The model under review builds one solid part; all positions refer to its coordinate system, in mm. A direction names the side the tool comes from. Round coordinates to 2 decimals unless told otherwise and drop trailing zeros. Loops run counter-clockwise (first coordinate to the right, second up) from the corner with the lowest first, then second, coordinate; pieces in that order, holes last. Notation, with made-up numbers: (15, 88.25) -> (61, 88.25) arc R17 cw to (61, 104.25) -> close; hole circle Ø10 at (36.25, 16.5). An arc over 180 degrees is marked (long way). Return JSON: item names as keys, results as strings. Group by question number.
```python
from build123d import *

# Parameters (mm, degrees)
SKETCH1_R           = 3.175
BOSS_EXTRUDE1_DEPTH = 5.842
FILLET1_R           = 6.35
FILLET2_R           = 12.7


with BuildPart() as part:
    # Sketch1 → Boss-Extrude1 (new body)
    with BuildSketch(Plane.XY):
        with BuildLine():
            Line((-22.994485403, 20.272024726), (-17.997254848, 15.918288597))
            Line((-17.997254848, 15.918288597), (-17.997254848, 5.482991472))
            Line((-17.997254848, 5.482991472), (-22.994485403, 1.145618131))
            ThreePointArc((-22.994485403, 1.145618131), (-24.602923257, -1.012071311), (-25.173214286, -3.642178571))
            ThreePointArc((-25.173214286, -3.642178571), (-21.763981419, -9.270178986), (-15.197028879, -8.854978145))
            Line((-15.197028879, -8.854978145), (-1.135121582, 0.926921642))
            Line((-1.135121582, 0.926921642), (26.988693011, 0.926921642))
            Line((26.988693011, 0.926921642), (42.638100307, -8.854978145))
            ThreePointArc((42.638100307, -8.854978145), (49.205052848, -9.270178986), (52.614285714, -3.642178571))
            ThreePointArc((52.614285714, -3.642178571), (52.043994686, -1.012071311), (50.435556832, 1.145618131))
            Line((50.435556832, 1.145618131), (46.348568334, 6.363266694))
            Line((46.348568334, 6.363266694), (46.348568334, 16.798563819))
            Line((46.348568334, 16.798563819), (50.435556832, 20.272024726))
            ThreePointArc((50.435556832, 20.272024726), (51.272005862, 28.964336626), (42.638100307, 30.272621002))
            Line((42.638100307, 30.272621002), (26.988693011, 20.490721215))
            Line((26.988693011, 20.490721215), (-1.135121582, 20.490721215))
            Line((-1.135121582, 20.490721215), (-15.197028879, 30.272621002))
            ThreePointArc((-15.197028879, 30.272621002), (-23.830934433, 28.964336626), (-22.994485403, 20.272024726))
        make_face()
        with Locations((-18.823214286, -3.642178571)):
            Circle(SKETCH1_R, mode=Mode.SUBTRACT)
        with Locations((46.264285714, -3.642178571)):
            Circle(SKETCH1_R, mode=Mode.SUBTRACT)
        with Locations((-18.823214286, 25.059821429)):
            Circle(SKETCH1_R, mode=Mode.SUBTRACT)
        with Locations((46.264285714, 25.059821429)):
            Circle(SKETCH1_R, mode=Mode.SUBTRACT)
    extrude(amount=BOSS_EXTRUDE1_DEPTH)

    # Fillet1
    fillet1_edges = [part.edges().sort_by_distance(p)[0] for p in [
        (-17.997254848, 5.482991472, 2.921),
        (-17.997254848, 15.918288597, 2.921),
        (46.348568334, 16.798563819, 2.921),
        (46.348568334, 6.363266694, 2.921),
    ]]
    fillet(fillet1_edges, radius=FILLET1_R)

    # Fillet2
    fillet2_edges = [part.edges().sort_by_distance(p)[0] for p in [
        (26.988693011, 0.926921642, 2.921),
        (-1.135121582, 0.926921642, 2.921),
        (-1.135121582, 20.490721215, 2.921),
        (26.988693011, 20.490721215, 2.921),
    ]]
    fillet(fillet2_edges, radius=FILLET2_R)


solid = part.part
```
1. For P1, Ø2, axis at y = 22, z = 2, coming from the +X side; P2, Ø3, axis at y = 21, z = 3, coming from the -X side; P3, Ø1.5, axis at x = 42.5, z = 1, coming from the +Y side, all flat-tipped, find the tip position at first contact; note any pin that passes through.
2. We need section C-C, the plane x = 13.5. Write out the cut boundary in (y, z).
3. We need section D-D, the plane y = 10.5. Write out the cut boundary in (x, z), then the cut area to 3 significant figures.
4. Tool access review of faces 1 (the face through (-18.58, 15.69, 2.96)), 2 (the face through (-9.73, 26.47, 2.88)), 3 (the face through (46.349, 11, 3)): name each direction out of +Z, -Z, +X, -X, +Y, -Y from which nothing blocks a thin tool from reaching the whole face with its end or side.
5. We need section B-B, the plane z = 1.15. Write out the cut boundary in (x, y) (3 decimals), then the cut area to 3 significant figures.
6. We need section A-A, the plane y = 26.5. Write out the cut boundary in (x, z).
7. Draft analysis for pull direction Y (two halves, no side actions). For faces 4 (the face through (36.27, -4.874, 2.88)), 5 (the face through (26.8, 20.97, 2.96)), 6 (the face through (-15.89, 23.84, 2.88)), state which applies: pulls with the +Y half, pulls with the -Y half, needs draft (parallel to the pull), parting line crosses it, or undercut.
8. Wall thickness on line 1 (Y direction, x = 47.5, z = 2.7); line 2 (X direction, y = 25, z = 2.4); line 3 (X direction, y = 13.5, z = 2.7): over which ranges is each line inside the solid? List them lowest first.
Check sheet entries:
{
 "1": {"P1": "stops at x = 52.27", "P2": "stops at x = -24.63", "P3": "stops at y = 30.65"},
 "2": {"outline": "(0.93, 0) -> (20.49, 0) -> (20.49, 5.84) -> (0.93, 5.84) -> close"},
 "3": {"outline": "(-18, 0) -> (46.35, 0) -> (46.35, 5.84) -> (-18, 5.84) -> close", "area": "376 mm²"},
 "4": {"face 1": "+Z, -Z, -X", "face 2": "+Z, -Z, +Y", "face 3": "+Z, -Z, +X"},
 "5": {"outline": "(-22.994, 1.146) arc R6.35 ccw to (-15.197, -8.855) -> (-4.405, -1.347) arc R12.7 cw to (2.848, 0.927) -> (23.346, 0.927) arc R12.7 cw to (30.078, -1.004) -> (42.638, -8.855) arc R6.35 ccw to (50.436, 1.146) -> (47.7, 4.638) arc R6.35 cw to (46.349, 8.554) -> (46.349, 13.862) arc R6.35 cw to (48.586, 18.7) -> (50.436, 20.272) arc R6.35 ccw to (42.638, 30.273) -> (30.078, 22.421) arc R12.7 cw to (23.346, 20.491) -> (2.848, 20.491) arc R12.7 cw to (-4.405, 22.765) -> (-15.197, 30.273) arc R6.35 ccw to (-22.994, 20.272) -> (-20.176, 17.816) arc R6.35 cw to (-17.997, 13.029) -> (-17.997, 8.38) arc R6.35 cw to (-20.185, 3.584) -> close; hole circle Ø6.35 at (-18.823, -3.642); hole circle Ø6.35 at (-18.823, 25.06); hole circle Ø6.35 at (46.264, -3.642); hole circle Ø6.35 at (46.264, 25.06)", "area": "1,860 mm²"},
 "6": {"outline": "(-25.01, 0) -> (-21.65, 0) -> (-21.65, 5.84) -> (-25.01, 5.84) -> close; (-15.99, 0) -> (-9.77, 0) -> (-9.77, 5.84) -> (-15.99, 5.84) -> close; (36.6, 0) -> (43.43, 0) -> (43.43, 5.84) -> (36.6, 5.84) -> close; (49.09, 0) -> (52.45, 0) -> (52.45, 5.84) -> (49.09, 5.84) -> close"},
 "7": {"face 4": "pulls with the -Y half", "face 5": "pulls with the +Y half", "face 6": "undercut"},
 "8": {"line 1": "y = -9.87 to -6.57, -0.72 to 4.91, 17.51 to 22.14, 27.98 to 31.29", "line 2": "x = -25.17 to -22, -15.65 to -7.62, 34.2 to 43.09, 49.44 to 52.61", "line 3": "x = -18.01 to 46.35"}
}
